from build123d import *

# Parameters (mm, degrees)
BASE_PLATE_PROFILE_DEPTH                     = 4.7625
M3_CLEARANCE_HOLE_FOR_CYLINDER_D             = 3.4
M3X0_5_TAPPED_HOLE_FOR_SUPPORT_PILLARS_D     = 2.5
M3X0_5_TAPPED_HOLE_FOR_SUPPORT_PILLARS_DEPTH = 7.5
M3X0_5_TAPPED_HOLE_FOR_SUPPORT_PILLARS_TIP   = 0.751075774
F_3_0MM_DOWEL_HOLE_FOR_SUPPORT_PILLARS_D     = 3
F_3_0MM_DOWEL_HOLE_FOR_SUPPORT_PILLARS_DEPTH = 6
F_3_0MM_DOWEL_HOLE_FOR_SUPPORT_PILLARS_TIP   = 0.901290929
M3X0_5_TAPPED_HOLE_FOR_PCB_STANDOFFS_D       = 2.5
M3X0_5_TAPPED_HOLE_FOR_PCB_STANDOFFS_DEPTH   = 6.5
M3X0_5_TAPPED_HOLE_FOR_PCB_STANDOFFS_TIP     = 0.751075774
M8_CLEARANCE_HOLE_FOR_LIFTING_ALIGNM_D       = 9
M8X1_25_TAPPED_HOLE_FOR_SUPER_STRUCTURE_D    = 6.8
F_7_16_20_TAPPED_HOLE_FOR_PENETRATOR_D       = 9.92124
SKETCH28_R                                   = 240.5
SKETCH28_R_2                                 = 236.3344
O_RING_GROOVE_DEPTH                          = 2.413
CIRPATTERN_EXTRACABLES_COUNT                 = 2
CIRPATTERN_EXTRACABLES_ANGLE                 = 15
F_5_8_CLEARANCE_HOLE1_D                      = 16.66748
SKETCH35_R                                   = 18
CUT_EXTRUDE1_DEPTH                           = 4.5
M8_CLEARANCE_HOLE_D                          = 9
F_5_0MM_DOWEL_HOLE1_D                        = 5.05
F_5_0MM_DOWEL_HOLE1_DEPTH                    = 5
F_5_0MM_DOWEL_HOLE1_TIP                      = 1.517173063


with BuildPart() as part:
    # Sketch1 → Base Plate Profile (new, symmetric)
    with BuildSketch(Plane(origin=(0, 0, 0), x_dir=(1, 0, 0), z_dir=(0, 1, 0))):
        Polygon((-131.979797464, 264), (131.979797464, 264), (264, 131.979797464), (264, -131.979797464), (131.979797464, -264), (-131.979797464, -264), (-264, -131.979797464), (-264, 131.979797464), align=None)
    extrude(amount=BASE_PLATE_PROFILE_DEPTH, both=True)

    # M3 Clearance Hole - For Cylinder (through all)
    with Locations(Plane(origin=(0, 4.7625, 0), x_dir=(1, 0, 0), z_dir=(0, 1, 0))):
        with Locations((248, 0), (243.23474954, -48.38239986), (229.122124063, -94.905491227), (206.204463851, -137.781417789), (175.362481734, -175.362481734), (137.781417789, -206.204463851), (94.905491227, -229.122124063), (48.38239986, -243.23474954), (0, -248), (-48.38239986, -243.23474954), (-94.905491227, -229.122124063), (-137.781417789, -206.204463851), (-175.362481734, -175.362481734), (-206.204463851, -137.781417789), (-229.122124063, -94.905491227), (-243.23474954, -48.38239986), (-248, 0), (-243.23474954, 48.38239986), (-229.122124063, 94.905491227), (-206.204463851, 137.781417789), (-175.362481734, 175.362481734), (-137.781417789, 206.204463851), (-94.905491227, 229.122124063), (-48.38239986, 243.23474954), (0, 248), (48.38239986, 243.23474954), (94.905491227, 229.122124063), (137.781417789, 206.204463851), (175.362481734, 175.362481734), (206.204463851, 137.781417789), (229.122124063, 94.905491227), (243.23474954, 48.38239986)):
            Hole(M3_CLEARANCE_HOLE_FOR_CYLINDER_D / 2)

    # M3x0.5 Tapped Hole - For Support Pillars
    with Locations(Plane(origin=(0, 4.7625, 0), x_dir=(1, 0, 0), z_dir=(0, 1, 0))):
        with Locations((-9, 201), (9, 201), (169.571106161, 108.294228634), (178.571106161, 92.705771366), (178.571106161, -92.705771366), (169.571106161, -108.294228634), (9, -201), (-9, -201), (-169.571106161, -108.294228634), (-178.571106161, -92.705771366), (-178.571106161, 92.705771366), (-169.571106161, 108.294228634)):
            Hole(M3X0_5_TAPPED_HOLE_FOR_SUPPORT_PILLARS_D / 2, depth=M3X0_5_TAPPED_HOLE_FOR_SUPPORT_PILLARS_DEPTH)
            with Locations((0, 0, -(M3X0_5_TAPPED_HOLE_FOR_SUPPORT_PILLARS_DEPTH + M3X0_5_TAPPED_HOLE_FOR_SUPPORT_PILLARS_TIP / 2))):  # 118° drill point
                Cone(0, M3X0_5_TAPPED_HOLE_FOR_SUPPORT_PILLARS_D / 2, M3X0_5_TAPPED_HOLE_FOR_SUPPORT_PILLARS_TIP, mode=Mode.SUBTRACT)

    # Ø3.0mm Dowel Hole - For Support Pillars
    with Locations(Plane(origin=(0, 4.7625, 0), x_dir=(1, 0, 0), z_dir=(0, 1, 0))):
        with Locations((9, 193), (-9, -193)):
            Hole(F_3_0MM_DOWEL_HOLE_FOR_SUPPORT_PILLARS_D / 2, depth=F_3_0MM_DOWEL_HOLE_FOR_SUPPORT_PILLARS_DEPTH)
            with Locations((0, 0, -(F_3_0MM_DOWEL_HOLE_FOR_SUPPORT_PILLARS_DEPTH + F_3_0MM_DOWEL_HOLE_FOR_SUPPORT_PILLARS_TIP / 2))):  # 118° drill point
                Cone(0, F_3_0MM_DOWEL_HOLE_FOR_SUPPORT_PILLARS_D / 2, F_3_0MM_DOWEL_HOLE_FOR_SUPPORT_PILLARS_TIP, mode=Mode.SUBTRACT)

    # M3x0.5 Tapped Hole - For PCB Standoffs
    with Locations(Plane(origin=(0, 4.7625, 0), x_dir=(1, 0, 0), z_dir=(0, 1, 0))):
        with Locations((113, 31), (-130, -130), (130, -130), (130, 130), (-130, 130), (-86.8, -86.7), (0, -122), (-123, -1), (-87.7, 85.8), (4, 27), (-2, 122)):
            Hole(M3X0_5_TAPPED_HOLE_FOR_PCB_STANDOFFS_D / 2, depth=M3X0_5_TAPPED_HOLE_FOR_PCB_STANDOFFS_DEPTH)
            with Locations((0, 0, -(M3X0_5_TAPPED_HOLE_FOR_PCB_STANDOFFS_DEPTH + M3X0_5_TAPPED_HOLE_FOR_PCB_STANDOFFS_TIP / 2))):  # 118° drill point
                Cone(0, M3X0_5_TAPPED_HOLE_FOR_PCB_STANDOFFS_D / 2, M3X0_5_TAPPED_HOLE_FOR_PCB_STANDOFFS_TIP, mode=Mode.SUBTRACT)

    # M8 Clearance Hole - For Lifting / Alignment (through all)
    with Locations(Plane(origin=(0, 4.7625, 0), x_dir=(1, 0, 0), z_dir=(0, 1, 0))):
        with Locations((-193.040151264, -193.040151264), (-193.040151264, 193.040151264), (193.040151264, 193.040151264), (193.040151264, -193.040151264)):
            Hole(M8_CLEARANCE_HOLE_FOR_LIFTING_ALIGNM_D / 2)

    # M8x1.25 Tapped Hole -For Super Structure (through all)
    with Locations(Plane(origin=(0, 4.7625, 0), x_dir=(1, 0, 0), z_dir=(0, 1, 0))):
        with Locations((250, 125), (-250, -125), (-250, 125), (250, -125)):
            Hole(M8X1_25_TAPPED_HOLE_FOR_SUPER_STRUCTURE_D / 2)

    # 7/16-20 Tapped Hole - For Penetrator (through all)
    with Locations(Plane(origin=(0, -4.7625, 0), x_dir=(-1, 0, 0), z_dir=(0, -1, 0))):
        with Locations((-200, 0)):
            f_7_16_20_tapped_hole_for_penetrator = Hole(F_7_16_20_TAPPED_HOLE_FOR_PENETRATOR_D / 2)

    # Sketch28 → O-ring Groove (cut)
    with BuildSketch(Plane(origin=(0, 4.7625, 0), x_dir=(1, 0, 0), z_dir=(0, 1, 0))):
        with Locations(Location((0, 0, 0), (0, 0, 270))):
            Circle(SKETCH28_R)
        with Locations(Location((0, 0, 0), (0, 0, 270))):
            Circle(SKETCH28_R_2, mode=Mode.SUBTRACT)
    extrude(amount=-O_RING_GROOVE_DEPTH, mode=Mode.SUBTRACT)

    # CirPattern_extraCables: 7/16-20 Tapped Hole - For Penetrator ×2 about axis
    cirpattern_extracables_axis = Axis((0, -5.23875, 0), (0, 1, 0))
    for i in range(1, CIRPATTERN_EXTRACABLES_COUNT):
        add(f_7_16_20_tapped_hole_for_penetrator.rotate(cirpattern_extracables_axis, i * CIRPATTERN_EXTRACABLES_ANGLE / (CIRPATTERN_EXTRACABLES_COUNT - 1)), mode=Mode.SUBTRACT)

    # 5/8 Clearance Hole1 (through all)
    with Locations(Plane(origin=(0, 4.7625, 0), x_dir=(1, 0, 0), z_dir=(0, 1, 0))):
        with Locations((193.185165258, -51.763809021)):
            Hole(F_5_8_CLEARANCE_HOLE1_D / 2)

    # Sketch35 → Cut-Extrude1 (cut)
    with BuildSketch(Plane.XZ.offset(4.7625)):
        with Locations(Location((193.185165258, 51.763809021, 0), (0, 0, 270))):
            Circle(SKETCH35_R)
    extrude(amount=-CUT_EXTRUDE1_DEPTH, mode=Mode.SUBTRACT)

    # M8 Clearance Hole (through all)
    with Locations(Plane(origin=(-28.123925909, 4.7625, -48.06749493), x_dir=(1, 0, 0), z_dir=(0, 1, 0))):
        with Locations((-96.876074091, -298.06749493), (-96.876074091, 201.93250507), (153.123925909, -298.06749493), (153.123925909, 201.93250507)):
            Hole(M8_CLEARANCE_HOLE_D / 2)

    # Ø5.0mm Dowel Hole1
    with Locations(Plane(origin=(0, 4.7625, 0), x_dir=(1, 0, 0), z_dir=(0, 1, 0))):
        with Locations((71.184478229, 236.520126119), (-71.184478229, -236.520126119)):
            Hole(F_5_0MM_DOWEL_HOLE1_D / 2, depth=F_5_0MM_DOWEL_HOLE1_DEPTH)
            with Locations((0, 0, -(F_5_0MM_DOWEL_HOLE1_DEPTH + F_5_0MM_DOWEL_HOLE1_TIP / 2))):  # 118° drill point
                Cone(0, F_5_0MM_DOWEL_HOLE1_D / 2, F_5_0MM_DOWEL_HOLE1_TIP, mode=Mode.SUBTRACT)


solid = part.part
The listing builds one solid part. Answer for the finished solid, in the listing's coordinates (mm). A direction names the side the tool comes from. Give positions to 0.01 mm unless a question says otherwise; leave off trailing zeros. One line per question, with ' | ' between items. Start each with the question number.
1. Straight lines are drawn through the part: line 1 (Z direction, x = 248, y = -0.25); line 2 (X direction, y = -2.75, z = -206.5); line 3 (Z direction, x = 55.5, y = 3.5). For each, find the intervals that lie inside material, in ascending order.
2. For faces 5 (the face through (211.03, -2.54, 54.11)), 6 (the face through (-159, 2.35, 177)), 7 (the face through (-198.91, 0.07, -197.07)), determine the directions among +Z, -Z, +X, -X, +Y, -Y from which every point of the face is accessible in a straight line to the end or side of a thin tool.
3. Given P1, Ø1.5, axis at x = -86.8, z = 86.7, coming from the +Y side; P2, Ø5, axis at x = -151.5, y = -2.5, coming from the -Z side, each flat-ended and moving along its own axis, determine where each tip first touches the part or whether it passes through.
4. Determine the mould class of faces 1 (the face through (72.24, 3.573, 229.394)), 2 (the face through (3, 4.762, -3)), 3 (the face through (-197.07, 0.07, 198.91)), 4 (the face through (185, -0.263, 48)) for opening direction X: +X half, -X half, draft (parallel to the pull), parting line (faces both ways), or undercut.
Result:
1) line 1: z = -147.98 to -127.75, -122.25 to -1.7, 1.7 to 122.25, 127.75 to 147.98 | line 2: x = -189.48 to -139.46, -136.11 to 136.11, 139.46 to 189.48 | line 3: z = -264 to -234.01, -229.73 to 229.73, 234.01 to 264
2) face 5: -Y | face 6: +Y | face 7: -Z, -X, +Y, -Y
3) P1: stops at y = -2.04 | P2: stops at z = -246.98
4) face 1: undercut | face 2: draft | face 3: -X half | face 4: undercut
